Check sheet for the modelled part. Datum: model origin and axes. Units: mm. A direction names the side the tool comes from. Coordinates: 2 decimals unless noted, no trailing zeros. Write each loop counter-clockwise with the first axis right and the second up, starting at its lowest first coordinate (ties: lowest second). Pieces come first, ordered by that corner, then holes. Notation, with made-up numbers: (-28, 49) -> (1, 49) arc R32 cw to (1, 88) -> close; hole circle Ø9 at (-31, -40). An arc over 180 degrees is marked (long way). Put each result on its own line as item: value.
```python
from build123d import *

# Parameters (mm, degrees)
PAD_DEPTH    = 2
SKETCH002_R  = 1.3
POCKET_DEPTH = 3.415102
PAD001_DEPTH = 1


with BuildPart() as part:
    # Sketch → Pad (new body)
    with BuildSketch(Plane.XY):
        with BuildLine():
            ThreePointArc((2, -3.464102), (0, 4), (-2, -3.464102))
            Line((-2, -6), (-2, -3.464102))
            Line((-2, -6), (-2, -8.535898))
            ThreePointArc((-2, -8.535898), (0, -16), (2, -8.535898))
            Line((2, -8.535898), (2, -6))
            Line((2, -3.464102), (2, -6))
        make_face()
        Polygon((0, 2.367136), (-2.05, 1.183568), (-2.05, -1.183568), (0, -2.367136), (2.05, -1.183568), (2.05, 1.183568), align=None, mode=Mode.SUBTRACT)
        Polygon((0, -14.367136), (-2.05, -13.183568), (-2.05, -10.816432), (0, -9.632864), (2.05, -10.816432), (2.05, -13.183568), align=None, mode=Mode.SUBTRACT)
    extrude(amount=PAD_DEPTH)

    # Sketch002 → Pocket (cut, through all)
    with BuildSketch(Plane(origin=(6.221152, -10.775352, 0), x_dir=(-0.866025, -0.5, 0), z_dir=(-0.5, 0.866025, 0))):
        Circle(SKETCH002_R)
    extrude(amount=-POCKET_DEPTH, mode=Mode.SUBTRACT)

    # Sketch003 → Pad001 (join)
    with BuildSketch(Plane.XY):
        with BuildLine():
            ThreePointArc((2, -3.464102), (0, 4), (-2, -3.464102))
            Line((-2, -6), (-2, -3.464102))
            Line((-2, -6), (-2, -8.535898))
            ThreePointArc((-2, -8.535898), (0, -16), (2, -8.535898))
            Line((2, -8.535898), (2, -6))
            Line((2, -3.464102), (2, -6))
        make_face()
    extrude(amount=-PAD001_DEPTH)


solid = part.part
```
Q1. Cross-section at B-B (z = 0.45). Record the cut outline in (x, y).
Recorded:
outline: (-2, -8.54) arc R4 ccw (long way) to (2, -8.54) -> (2, -3.46) arc R4 ccw (long way) to (-2, -3.46) -> close; hole (-2.05, -13.18) -> (0, -14.37) -> (2.05, -13.18) -> (2.05, -10.82) -> (0, -9.63) -> (-2.05, -10.82) -> close; hole (-2.05, -1.18) -> (0, -2.37) -> (2.05, -1.18) -> (2.05, 1.18) -> (0, 2.37) -> (-2.05, 1.18) -> close
Q2. Material ranges on line 1 along Y through (x, z) = (0.75, 1.5); line 2 along Y through (x, z) = (-1.5, 0.4); line 3 along Z through (x, y) = (0, -13), recorded low to high.
Recorded:
line 1: y = -15.93 to -13.93, -10.07 to -1.93, 1.93 to 3.93
line 2: y = -15.71 to -13.5, -10.5 to -1.5, 1.5 to 3.71
line 3: z = -1 to 0
Q3. Tool access check on faces 1 (the flat face through (2, -6, 1)), 2 (the flat face through (0, -6, -1)), 3 (the flat face through (0, -12, 0)). Record the directions out of +Z, -Z, +X, -X, +Y, -Y that give a thin tool (end or side, any length) a straight path to the whole face; none if there is none.
Recorded:
face 1: +Z, -Z, +X
face 2: -Z, +X, -X, +Y, -Y
face 3: +Z
Q4. Cross-section at D-D (x = -1.25). Record the cut outline in (y, z).
Recorded:
outline: (-15.8, -1) -> (3.8, -1) -> (3.8, 2) -> (1.65, 2) -> (1.65, 0) -> (-1.65, 0) -> (-1.65, 2) -> (-10.35, 2) -> (-10.35, 0) -> (-13.65, 0) -> (-13.65, 2) -> (-15.8, 2) -> close
Q5. Cross-section at C-C (x = -2.25). Record the cut outline in (y, z).
Recorded:
outline: (-15.31, -1) -> (-8.69, -1) -> (-8.69, 2) -> (-15.31, 2) -> close; (-3.31, -1) -> (3.31, -1) -> (3.31, 2) -> (-3.31, 2) -> close
Q6. Mould release check, pull along X, two halves, no side actions. Record for faces 4 (the flat face through (1.039, -13.767, 0.986)), 5 (the flat face through (0, -6, 2)), 6 (the flat face through (-2, -6, 1)): released by +X, released by -X, zero draft, split by the parting line, or undercut.
Recorded:
face 4: undercut
face 5: zero draft
face 6: released by -X
Q7. Depth check by flat-ended pin: P1, Ø0.6, axis at y = -12.5, z = 1, coming from the -X side (3 decimals). Enter the tip coordinate at first touch or a pass-through.
Recorded:
P1: stops at x = -3.995
Q8. Cross-section at A-A (y = 0). Record the cut outline in (x, z), plus the area to 3 significant figures.
Recorded:
outline: (-4, -1) -> (4, -1) -> (4, 2) -> (2.05, 2) -> (2.05, 0) -> (-2.05, 0) -> (-2.05, 2) -> (-4, 2) -> close
area: 15.8 mm2
